Could you check a few things on this drawing? It's one solid part, dimensions in mm from its lowest x, y, z. A direction names the side the tool comes from. Give positions to 0.01 mm unless a question says otherwise; leave off trailing zeros. Order: outer loops, then holes, each group sorted by start corner. A loop starts at its lowest first (then second) coordinate and runs counter-clockwise, first axis right, second up.
Item 1: I want a section at C-C, the plane z = 5.15. Write out the boundary of the cut face in (x, y).
Item 2: I want a section at D-D, the plane y = 1.5. Write out the boundary of the cut face in (x, z), then the cut area to 3 significant figures.
Item 3: I'm going to push flat-ended pins straight in: pin 1 Ø1.2 at (x, y) = (4.5, 5) entering from +Z; pin 2 Ø4 at (x, y) = (10.5, 3) entering from -Z. Where does each tip first touch, or does it pass through?
Item 4: Which directions (+Z, -Z, +X, -X, +Y, -Y) give clear straight access to the entire face, cutting with the end or side of a thin tool? Please do the marked faces 4 and 5.
Item 5: If I drill on line 1 along X through (y, z) = (2.85, 3); line 2 along Y through (x, z) = (11.5, 2); line 3 along X through (y, z) = (5.5, 4.5), over which ranges is the centre line in solid material (lowest first)?
Item 6: If we mould it in two halves opening along Y, with no side actions, what happens to the marked faces 1, 2 and 3? For each: +Y half, -Y half, draft (parallel to the pull), parting line (faces both ways), or undercut.
Item 7: I want a section at B-B, the plane x = 11.5. Write out the boundary of the cut face in (y, z).
Item 8: I want a section at A-A, the plane y = 4.25. Write out the boundary of the cut face in (x, z).
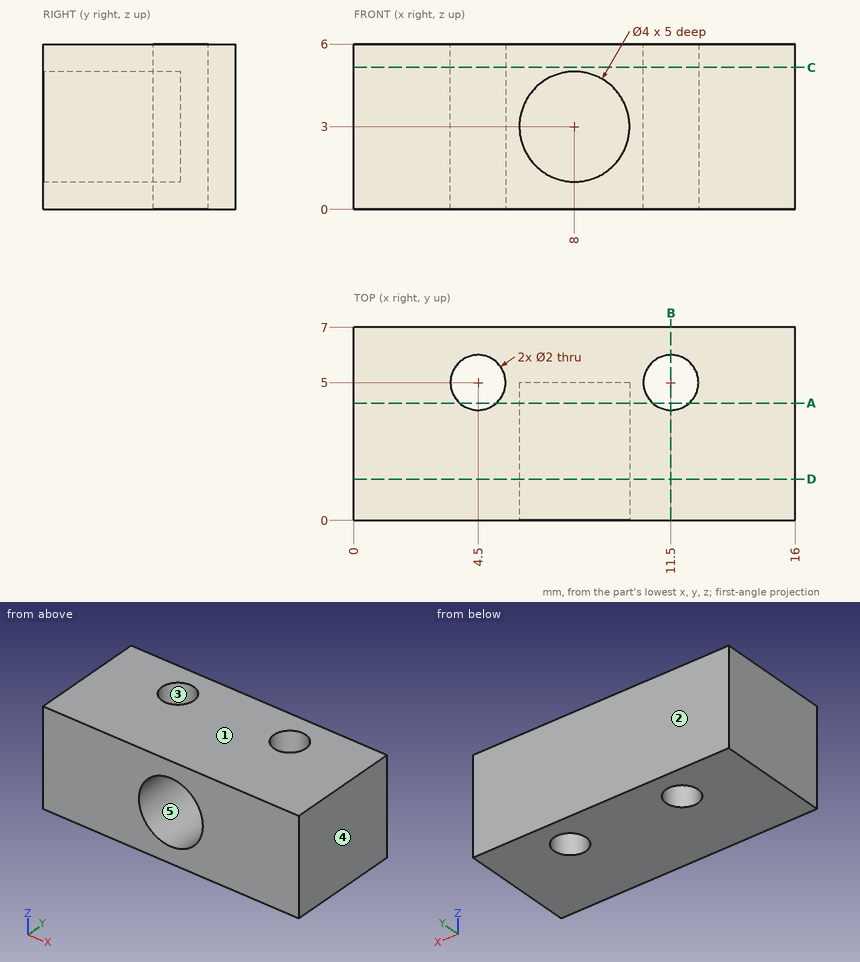
Results list:
1. outline: (0, 0) - (16, 0) - (16, 7) - (0, 7) - close; hole circle Ø2 at (4.5, 5); hole circle Ø2 at (11.5, 5)
2. outline: (0, 0) - (16, 0) - (16, 6) - (0, 6) - close; hole circle Ø4 at (8, 3)
2. area: 83.4 mm2
3. pin 1: passes through
3. pin 2: stops at z = 0
4. face 4: +Z, -Z, +X, +Y, -Y
4. face 5: -Y
5. line 1: x = 0 to 6, 10 to 16
5. line 2: y = 0 to 4, 6 to 7
5. line 3: x = 0 to 3.63, 5.37 to 10.63, 12.37 to 16
6. face 1: draft
6. face 2: +Y half
6. face 3: undercut
7. outline: (0, 0) - (4, 0) - (4, 6) - (0, 6) - close; (6, 0) - (7, 0) - (7, 6) - (6, 6) - close
8. outline: (0, 0) - (3.84, 0) - (3.84, 6) - (0, 6) - close; (5.16, 0) - (10.84, 0) - (10.84, 6) - (5.16, 6) - close; (12.16, 0) - (16, 0) - (16, 6) - (12.16, 6) - close; hole circle Ø4 at (8, 3)
